```python
from build123d import *

# Parameters (mm, degrees)
PAD_DEPTH    = 1.5
PAD001_DEPTH = 1.5
FILLET_R     = 0.3
FILLET001_R  = 0.3


with BuildPart() as part:
    # Sketch → Pad (new body)
    with BuildSketch(Plane.XY):
        with BuildLine():
            ThreePointArc((-3.805944, 5.269231), (2, -6.184658), (0, 6.5))
            Line((0, 6.5), (0, 5))
            ThreePointArc((-2.927649, 4.053254), (1.538462, -4.75743), (0, 5))
            Line((-3.805944, 5.269231), (-2.927649, 4.053254))
        make_face()
    extrude(amount=PAD_DEPTH)

    # Sketch001 (on Face6 of Pad) → Pad001 (join)
    with BuildSketch(Plane.XY):
        with BuildLine():
            ThreePointArc((-2.927649, 4.053254), (1.538462, -4.75743), (0, 5))
            Line((0, 7), (0, 5))
            ThreePointArc((-4.098709, 5.674556), (2.153846, -6.660401), (0, 7))
            Line((-4.098709, 5.674556), (-2.927649, 4.053254))
        make_face()
    extrude(amount=-PAD001_DEPTH)

    # Fillet
    fillet_edges = [part.edges().sort_by_distance(p)[0] for p in [
        (1.538462, -4.75743, 1.5),
    ]]
    fillet(fillet_edges, radius=FILLET_R)

    # Fillet001
    fillet001_edges = [part.edges().sort_by_distance(p)[0] for p in [
        (1.538462, -4.75743, -1.5),
    ]]
    fillet(fillet001_edges, radius=FILLET001_R)


solid = part.part
```
Source: CAD feature listing. Evaluate the final solid. Frame: model axes, mm. A direction names the side the tool comes from. Round coordinates to 2 decimals unless told otherwise and drop trailing zeros. Loops run counter-clockwise (first coordinate to the right, second up) from the corner with the lowest first, then second, coordinate; pieces in that order, holes last.
1. Ray query, L1, parallel to X at y = 0, z = -0.4; L2, parallel to X at y = 0, z = 0.2; L3, parallel to Y at x = 2, z = 0.2. Return the intervals inside material, ascending.
2. Contact query for a flat-ended pin moving along its axis: pin 1 (6 mm diameter, centred on x = -0.5, y = -2.5, fed in from +Z). Output: stop coordinate, or through.
3. Mould query, pull axis Y, two halves, no side actions, for faces 1 (the cylindrical face through (1.349, -4.815, 0.017)), 2 (the flat face through (4, -4, -1.5)), 3 (the cylindrical face through (1.75, -6.26, 0.74)). Classes: released by +Y, released by -Y, zero draft, split by the parting line, or undercut.
4. Access query for faces 4 (the cylindrical face through (1.89, -6.74, -0.74)), 5 (the flat face through (0, -6.7, 0)), 6 (the flat face through (0, 6, 0)). Directions: +Z, -Z, +X, -X, +Y, -Y. A direction counts if a zero-diameter tool reaches every point of the face in a straight line with its end or side. Return the directions, or none.
5. Section query A-A on x = 6. Output: boundary loops of the cut face in (y, z).
6. Section query C-C on z = -0.75. Output: boundary loops of the cut face in (x, y).
Answers below:
1. L1: x = -7 to -5, 5 to 7
1. L2: x = -6.5 to -5, 5 to 6.5
1. L3: y = -6.18 to -4.58, 4.58 to 6.18
2. pin 1: stops at z = 1.5
3. face 1: undercut
3. face 2: zero draft
3. face 3: split by the parting line
4. face 4: +Z, -Z
4. face 5: +Z
4. face 6: +Z, -Z, +Y
5. outline: (-3.61, -1.5) - (3.61, -1.5) - (3.61, 0) - (2.5, 0) - (2.5, 1.5) - (-2.5, 1.5) - (-2.5, 0) - (-3.61, 0) - close
6. outline: (-4.1, 5.67) arc R7 ccw (long way) to (0, 7) - (0, 5) arc R5 cw (long way) to (-2.93, 4.05) - close
